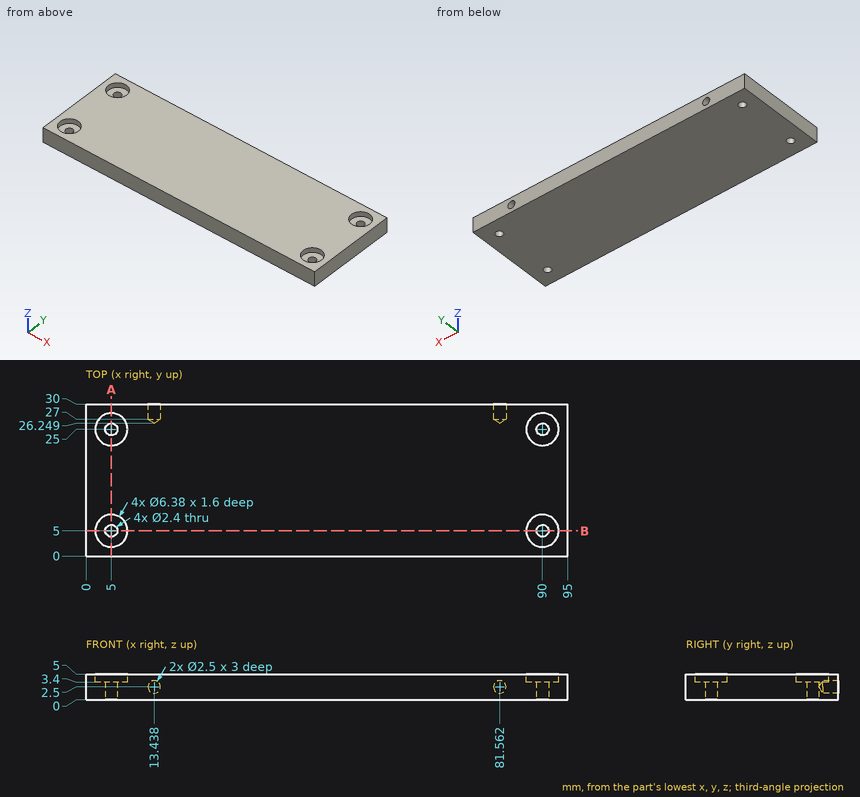
Geometry check sheet. Reference: drawing and pictorial views, mm from the part's lowest x, y, z. Give positions to 0.01 mm unless a question says otherwise; leave off trailing zeros. Order: outer loops, then holes, each group sorted by start corner. A loop starts at its lowest first (then second) coordinate and runs counter-clockwise, first axis right, second up. Notation, with made-up numbers: M 10.5,17 L 41.5,17 A18 ccw 41.5,51 Z; hole C 83,67.25 d9. An arc over 180 degrees is marked long. Answer in a Markdown table with one row per item. Add a question column.
Item 1: Section check B-B, the plane y = 5. Enter the section's corners in (x, z), and give its area (3 significant figures).
Item 2: Scan lines: probe 1 along Y at (x, z) = (5, 3.8); probe 2 along X at (y, z) = (27.25, 4.5); probe 3 along Y at (x, z) = (91.5, 3.9) (1 decimal). Record each from-to range of solid material in increasing order. Write a range as from..to.
Item 3: Gauge pin test, flat ends, axial feed: pin 1 (4 mm diameter, centred on x = 5, y = 5, fed in from +Z); pin 2 (2 mm diameter, centred on x = 81.56, z = 2.5, fed in from +Y). Record the tip position at first contact, or that the pin passes through.
Item 4: Section check A-A, the plane x = 5. Enter the section's corners in (y, z).
Filled sheet:
| question | item | result |
|---|---|---|
| 1 | outline | M 0,0 L 3.8,0 L 3.8,3.4 L 1.81,3.4 L 1.81,5 L 0,5 Z; M 6.2,0 L 88.8,0 L 88.8,3.4 L 86.81,3.4 L 86.81,5 L 8.19,5 L 8.19,3.4 L 6.2,3.4 Z; M 91.2,0 L 95,0 L 95,5 L 93.19,5 L 93.19,3.4 L 91.2,3.4 Z |
| 1 | area | 438 mm^2 |
| 2 | probe 1 | y = 0..1.81, 8.19..21.81, 28.19..30 |
| 2 | probe 2 | x = 0..2.74, 7.26..87.74, 92.26..95 |
| 2 | probe 3 | y = 0..2.2, 7.8..22.2, 27.8..30 |
| 3 | pin 1 | stops at z = 3.4 |
| 3 | pin 2 | stops at y = 26.85 |
| 4 | outline | M 0,0 L 3.8,0 L 3.8,3.4 L 1.81,3.4 L 1.81,5 L 0,5 Z; M 6.2,0 L 23.8,0 L 23.8,3.4 L 21.81,3.4 L 21.81,5 L 8.19,5 L 8.19,3.4 L 6.2,3.4 Z; M 26.2,0 L 30,0 L 30,5 L 28.19,5 L 28.19,3.4 L 26.2,3.4 Z |
